from build123d import *

# Parameters (mm, degrees)
BOSS_EXTRUDE1_DEPTH = 110
CUT_EXTRUDE1_DEPTH  = 109.3
SKETCH3_R           = 3.375
CUT_EXTRUDE2_DEPTH  = 5
SKETCH4_W           = 40.6
SKETCH4_H           = 19.3
CUT_EXTRUDE3_DEPTH  = 15
FILLET1_R           = 3


with BuildPart() as part:
    # Sketch1 → Boss-Extrude1 (new body)
    with BuildSketch(Plane(origin=(0, 0, 0), x_dir=(1, 0, 0), z_dir=(0, 1, 0))):
        with BuildLine():
            Line((-40.883093525, -1.707733813), (1.116906475, -1.707733813))
            Line((1.116906475, -1.707733813), (1.116906475, 18.292266187))
            ThreePointArc((1.116906475, 18.292266187), (-19.883093525, 39.292266187), (-40.883093525, 18.292266187))
            Line((-40.883093525, 18.292266187), (-40.883093525, -1.707733813))
        make_face()
    extrude(amount=BOSS_EXTRUDE1_DEPTH)

    # Sketch2 → Cut-Extrude1 (cut)
    with BuildSketch(Plane(origin=(0, 110, 0), x_dir=(1, 0, 0), z_dir=(0, 1, 0))):
        with BuildLine():
            Line((-40.183093525, 16.292266187), (-40.183093525, 11.292266187))
            Line((-40.183093525, 11.292266187), (-34.183093525, 11.292266187))
            Line((-34.183093525, 11.292266187), (-34.183093525, 9.292266187))
            Line((-34.183093525, 9.292266187), (-40.183093525, 9.292266187))
            Line((-40.183093525, 9.292266187), (-40.183093525, -1.007733813))
            Line((-40.183093525, -1.007733813), (0.416906475, -1.007733813))
            Line((0.416906475, -1.007733813), (0.416906475, 9.292266187))
            Line((0.416906475, 9.292266187), (-5.583093525, 9.292266187))
            Line((-5.583093525, 9.292266187), (-5.583093525, 11.292266187))
            Line((-5.583093525, 11.292266187), (0.416906475, 11.292266187))
            Line((0.416906475, 11.292266187), (0.416906475, 16.292266187))
            Line((0.416906475, 16.292266187), (-5.583093525, 16.292266187))
            Line((-5.583093525, 16.292266187), (-5.583093525, 18.292266187))
            Line((-5.583093525, 18.292266187), (0.416906475, 18.292266187))
            ThreePointArc((0.416906475, 18.292266187), (-19.883093525, 38.592266187), (-40.183093525, 18.292266187))
            Line((-40.183093525, 18.292266187), (-34.183093525, 18.292266187))
            Line((-34.183093525, 18.292266187), (-34.183093525, 16.292266187))
            Line((-34.183093525, 16.292266187), (-40.183093525, 16.292266187))
        make_face()
    extrude(amount=-CUT_EXTRUDE1_DEPTH, mode=Mode.SUBTRACT)

    # Sketch3 → Cut-Extrude2 (cut)
    with BuildSketch(Plane.ZY.offset(40.883093525)):
        with Locations((-4.958932854, 55)):
            Circle(SKETCH3_R)
    extrude(amount=-CUT_EXTRUDE2_DEPTH, mode=Mode.SUBTRACT)

    # Sketch4 → Cut-Extrude3 (cut)
    with BuildSketch(Plane(origin=(0, 110, 0), x_dir=(1, 0, 0), z_dir=(0, 1, 0))):
        with Locations((-19.883093525, 8.642266187)):
            Rectangle(SKETCH4_W, SKETCH4_H)
    extrude(amount=-CUT_EXTRUDE3_DEPTH, mode=Mode.SUBTRACT)

    # Fillet1
    fillet1_edges = [part.edges().sort_by_distance(p)[0] for p in [
        (-40.183093525, 95, -17.292266187),
    ]]
    fillet(fillet1_edges, radius=FILLET1_R)
    fillet1_2_edges = [part.edges().sort_by_distance(p)[0] for p in [
        (-40.183093525, 95, -10.292266187),
    ]]
    fillet(fillet1_2_edges, radius=FILLET1_R)
    fillet1_3_edges = [part.edges().sort_by_distance(p)[0] for p in [
        (0.416906475, 95, -10.292266187),
    ]]
    fillet(fillet1_3_edges, radius=FILLET1_R)
    fillet1_4_edges = [part.edges().sort_by_distance(p)[0] for p in [
        (0.416906475, 95, -17.292266187),
    ]]
    fillet(fillet1_4_edges, radius=FILLET1_R)
    fillet1_5_edges = [part.edges().sort_by_distance(p)[0] for p in [
        (-5.583093525, 95, -17.292266187),
    ]]
    fillet(fillet1_5_edges, radius=FILLET1_R - 0.0001)  # a hair under: the kernel refuses the full size
    fillet1_6_edges = [part.edges().sort_by_distance(p)[0] for p in [
        (-5.583093525, 95, -10.292266187),
    ]]
    fillet(fillet1_6_edges, radius=FILLET1_R - 0.0001)  # a hair under: the kernel refuses the full size
    fillet1_7_edges = [part.edges().sort_by_distance(p)[0] for p in [
        (-34.183093525, 95, -10.292266187),
    ]]
    fillet(fillet1_7_edges, radius=FILLET1_R - 0.0001)  # a hair under: the kernel refuses the full size
    fillet1_8_edges = [part.edges().sort_by_distance(p)[0] for p in [
        (-34.183093525, 95, -17.292266187),
    ]]
    fillet(fillet1_8_edges, radius=FILLET1_R - 0.0001)  # a hair under: the kernel refuses the full size


solid = part.part
CAD build for the part. Positions are in the model's coordinates, mm. A direction names the side the tool comes from. Round coordinates to 2 decimals unless told otherwise and drop trailing zeros. Write each loop counter-clockwise with the first axis right and the second up, starting at its lowest first coordinate (ties: lowest second). Pieces come first, ordered by that corner, then holes. Notation, with made-up numbers: M 42,6 L 57,6 A21 cw 57,32 Z; hole C 8.25,-14.5 d1. An arc over 180 degrees is marked long. Use a Markdown table: item, result. Add a question column.
1. Drill centre lines: probe 1 along X at (y, z) = (70, -14); probe 2 along X at (y, z) = (62, -11); probe 3 along Y at (x, z) = (-18.5, -37). Where is each one in solid material? Low to high.
2. Flat gauge pins, fed straight in: P1, Ø8, axis at x = -21, z = -20.5, coming from the +Y side; P2, Ø2, axis at y = 16.5, z = -24.5, coming from the +X side; P3, Ø3, axis at x = -36.5, y = 30.5, coming from the -Z side. Where does each tip first touch, or does it go through?
3. Slice it at B-B on z = -21. Give the cut face in (x, y).
4. Slice it at C-C on y = 55. Give the cut face in (x, z), then the cut area to 3 significant figures.
5. Slice it at A-A on y = 80.5. Give the cut face in (x, z).
6. Slice it at D-D on x = -25.5. Give the cut face in (y, z), then the cut area to 3 significant figures.
7. 3-axis set-ups, long thin cutter, end or side, ignore diameter. For faces 4 (the face through (-39, 110, -26)), 5 (the face through (-3, 50, -11.292)), 6 (the face through (-40.538, 51.705, -5.691)): which of +Z, -Z, +X, -X, +Y, -Y reach the whole face in a straight line?
8. Pull direction X, two halves, no side cores. Call faces 1 (the face through (-20, 54, 1.708)), 2 (the face through (-37, 50, -9.292)), 3 (the face through (1.117, 54, -8)): released by +X, released by -X, zero draft, split by the parting line, or undercut.
Reply:
| question | item | result |
|---|---|---|
| 1 | probe 1 | x = -40.88 to -40.18, 0.42 to 1.12 |
| 1 | probe 2 | x = -40.88 to -34.18, -5.58 to 1.12 |
| 1 | probe 3 | y = 0 to 0.7 |
| 2 | P1 | stops at y = 0.7 |
| 2 | P2 | stops at x = 0.46 |
| 2 | P3 | stops at z = -32.87 |
| 3 | outline | M -40.71,0 L 0.94,0 L 0.94,110 L 0.24,110 L 0.24,0.7 L -40,0.7 L -40,110 L -40.71,110 Z |
| 4 | outline | M -40.88,-18.29 A21 ccw 1.12,-18.29 L 1.12,1.71 L -40.88,1.71 L -40.88,-1.58 L -40.18,-1.58 L -40.18,1.01 L 0.42,1.01 L 0.42,-9.29 L -5.58,-9.29 L -5.58,-11.29 L 0.42,-11.29 L 0.42,-16.29 L -5.58,-16.29 L -5.58,-18.29 L 0.42,-18.29 A20.3 cw -40.18,-18.29 L -34.18,-18.29 L -34.18,-16.29 L -40.18,-16.29 L -40.18,-11.29 L -34.18,-11.29 L -34.18,-9.29 L -40.18,-9.29 L -40.18,-8.33 L -40.88,-8.33 Z |
| 4 | area | 145 mm^2 |
| 5 | outline | M -40.88,-18.29 A21 ccw 1.12,-18.29 L 1.12,1.71 L -40.88,1.71 Z; hole M -40.18,-18.29 A20.3 ccw 0.42,-18.29 L -5.58,-18.29 L -5.58,-16.29 L 0.42,-16.29 L 0.42,-11.29 L -5.58,-11.29 L -5.58,-9.29 L 0.42,-9.29 L 0.42,1.01 L -40.18,1.01 L -40.18,-9.29 L -34.18,-9.29 L -34.18,-11.29 L -40.18,-11.29 L -40.18,-16.29 L -34.18,-16.29 L -34.18,-18.29 Z |
| 6 | outline | M 0,-38.53 L 110,-38.53 L 110,-37.8 L 0.7,-37.8 L 0.7,1.01 L 110,1.01 L 110,1.71 L 0,1.71 Z |
| 6 | area | 184 mm^2 |
| 7 | face 4 | +Z, -Z, +X, -X, +Y |
| 7 | face 5 | +Y |
| 7 | face 6 | -X |
| 8 | face 1 | zero draft |
| 8 | face 2 | undercut |
| 8 | face 3 | released by +X |
